Here's how the part is built. I have some questions about the finished solid (model axes, mm). A direction names the side the tool comes from. Give positions to 0.01 mm unless a question says otherwise; leave off trailing zeros. Loops run counter-clockwise (first coordinate to the right, second up) from the corner with the lowest first, then second, coordinate; pieces in that order, holes last. Notation, with made-up numbers: (42, 74) - (87, 74) arc R29 ccw to (87, 112) - close; hole circle Ø2 at (31.25, 61). An arc over 180 degrees is marked (long way). Return JSON: item names as keys, results as strings. Group by question number.
(1) If we section it at A-A (x = -38.5): Please give me the cut outline in (y, z), then the cut area to 3 significant figures.
(2) If we mould it in two halves opening along X, with no side actions, what happens to faces 1 (the flat face through (-19, 17, -96)), 2 (the flat face through (-140, 10, -94)), 3 (the flat face through (-69, 17, -11.5)), 4 (the flat face through (-130, -3, -95))? For each: released by +X, released by -X, zero draft, split by the parting line, or undercut.
(3) For P1, Ø1.5, axis at y = -1.5, z = -88, coming from the +X side; P2, Ø1.8, axis at x = -135, z = -5, coming from the -Y side; P3, Ø5, axis at x = -120.5, z = -8, coming from the -Y side; P4, Ø1.5, axis at y = -1.5, z = -110, coming from the -X side, each with a flat end and sliding along its axis, tell me the tip position at first contact or that it passes through.
(4) If we section it at C-C (y = 5.5): Please give me the cut outline in (x, z).
(5) I need wall thicknesses on probe 1 along X at (y, z) = (6, -5); probe 2 along Z at (x, y) = (-5, 4.25); probe 3 along X at (y, z) = (14.75, -5). Which ranges of each line are inside material? Lowest first, please. Write a range as [from, to].
(6) On a 3-axis mill with a long thin cutter (end or side, diameter ignored), from which of +Z, -Z, +X, -X, +Y, -Y can I reach the whole of each face in a straight line? I mean faces 5 (the flat face through (-71, 6, -185.4)), 6 (the flat face through (-121, 17, -94)), 7 (the flat face through (-133, -1, -183)). Say none if no direction works.
(7) If we section it at B-B (z = -138): Please give me the cut outline in (x, y).
Autodesk Inventor part; units mm, degrees
ref_plane "YZ Plane" through (0, 0, 0) normal (1, 0, 0) x (0, 1, 0)
ref_plane "XZ Plane" through (0, 0, 0) normal (0, 1, 0) x (-1, 0, 0)
ref_plane "XY Plane" through (0, 0, 0) normal (0, 0, 1) x (1, 0, 0)
sketch "Sketch1" plane through (0, 0, 0) normal (0, 1, 0) x (-1, 0, 0)
  line L0 (2, 0) -> (138, 0)
  line L1 (140, -2) -> (140, -188)
  line L2 (138, -190) -> (2, -190)
  line L3 (0, -188) -> (0, -2)
  arc A0 (140, -2) -> (138, 0) centre (138, -2) ccw
  arc A1 (2, 0) -> (0, -2) centre (2, -2) ccw
  arc A2 (0, -188) -> (2, -190) centre (2, -188) ccw
  arc A3 (138, -190) -> (140, -188) centre (138, -188) ccw
  line L4 (21, -11.5) -> (119, -11.5)
  line L5 (121, -13.5) -> (121, -176.5)
  line L6 (119, -178.5) -> (21, -178.5)
  line L7 (19, -176.5) -> (19, -13.5)
  arc A4 (121, -13.5) -> (119, -11.5) centre (119, -13.5) ccw
  arc A5 (119, -178.5) -> (121, -176.5) centre (119, -176.5) ccw
  arc A6 (19, -176.5) -> (21, -178.5) centre (21, -176.5) ccw
  arc A7 (21, -11.5) -> (19, -13.5) centre (21, -13.5) ccw
  point P0 (0, 0)
  point P1 (140, -190)
  point P2 (140, 0)
  point P3 (0, -190)
  point P4 (121, -178.5)
  point P5 (121, -11.5)
  point P6 (19, -178.5)
  dimension "d5" = 190
  dimension "d6" = 140
  dimension "d7" = 102
  dimension "d8" = 167
  dimension "d9" = 2
  dimension "d57" = 11.5
  dimension "d58" = 19
extrude "Extrusion1" add sketch "Sketch1" along normal blind 20
sketch "Sketch2" plane through (0, 0, 0) normal (0, -1, 0) x (1, 0, 0)
  line L0 (-11, -3) -> (-129, -3)
  line L1 (-137, -11) -> (-137, -179)
  line L2 (-129, -187) -> (-11, -187)
  line L3 (-3, -179) -> (-3, -11)
  line L4 (-137, -179) -> (-129, -187)
  line L5 (-137, -11) -> (-129, -3)
  line L6 (-11, -3) -> (-3, -11)
  line L7 (-11, -187) -> (-3, -179)
  line L8 (-129, -187) -> (-129, -185.4)
  line L9 (-129, -185.4) -> (-11, -185.4)
  line L10 (-11, -185.4) -> (-11, -4.6)
  line L11 (-11, -4.6) -> (-129, -4.6)
  line L12 (-129, -4.6) -> (-129, -185.4)
  point P0 (0, 0)
  point P1 (-3, -3)
  point P2 (-137, -187)
  point P3 (-137, -3)
  point P4 (-3, -187)
  dimension "d86" = 134
  dimension "d87" = 184
  dimension "d88" = 8
  dimension "d89" = 8
  dimension "d90" = 8
  dimension "d91" = 8
  dimension "d92" = 8
  dimension "d93" = 8
  dimension "d94" = 8
  dimension "d95" = 8
  dimension "d96" = 1.6
  dimension "d97" = 180.8
  dimension "d98" = 180.8
extrude "Extrusion2" add sketch "Sketch2" along normal blind 3
hole "Hole1" at (-135, 20, -5) direction (0, -1, 0) diameter 3 end through all countersink diameter 5 countersink angle 90
hole "Hole2" at (-135, 20, -185) direction (0, -1, 0) diameter 3 end through all countersink diameter 5 countersink angle 90
hole "Hole3" at (-5, 20, -185) direction (0, -1, 0) diameter 3 end through all countersink diameter 5 countersink angle 90
hole "Hole4" at (-5, 20, -5) direction (0, -1, 0) diameter 3 end through all countersink diameter 5 countersink angle 90
hole "Hole5" at (-120.5, 0, -8) direction (0, 1, 0) diameter 3 depth 19 tip angle 118
hole "Hole6" at (-19.5, 0, -8) direction (0, 1, 0) diameter 3 depth 19 tip angle 118
hole "Hole7" at (-120.5, 0, -182) direction (0, 1, 0) diameter 3 depth 19 tip angle 118
hole "Hole8" at (-19.5, 0, -182) direction (0, 1, 0) diameter 3 depth 19 tip angle 118
sketch "Sketch3" plane through (0, 0, 0) normal (0, -1, 0) x (1, 0, 0)
  line L0 (-11, -185.4) -> (-11, -4.6)
  line L1 (-129, -4.6) -> (-11, -4.6)
  line L2 (-11, -185.4) -> (-129, -185.4)
  line L3 (-129, -185.4) -> (-129, -4.6)
  line L4 (-129, -4.6) -> (-11, -4.6)
  line L5 (-11, -4.6) -> (-11, -185.4)
  point P0 (0, 0)
extrude "Extrusion3" cut sketch "Sketch3" against normal blind 14
properties part number "Dessus boitier"
Values:
{
 "1": {"outline": "(-3, -187) - (0, -187) - (0, -190) - (20, -190) - (20, -178.5) - (14, -178.5) - (14, -185.4) - (-3, -185.4) - close; (-3, -4.6) - (14, -4.6) - (14, -11.5) - (20, -11.5) - (20, 0) - (0, 0) - (0, -3) - (-3, -3) - close", "area": "276 mm2"},
 "2": {"face 1": "undercut", "face 2": "released by -X", "face 3": "undercut", "face 4": "zero draft"},
 "3": {"P1": "x = -3", "P2": "through", "P3": "y = 14", "P4": "x = -137"},
 "4": {"outline": "(-140, -188) arc R2 ccw to (-138, -190) - (-2, -190) arc R2 ccw to (0, -188) - (0, -2) arc R2 ccw to (-2, 0) - (-138, 0) arc R2 ccw to (-140, -2) - close; hole circle Ø3 at (-135, -185); hole circle Ø3 at (-135, -5); hole (-129, -185.4) - (-11, -185.4) - (-11, -4.6) - (-129, -4.6) - close; hole circle Ø3 at (-5, -185); hole circle Ø3 at (-5, -5)"},
 "5": {"probe 1": "[-140, -136.5], [-133.5, -129], [-11, -6.5], [-3.5, 0]", "probe 2": "[-190, -186.5], [-183.5, -6.5], [-3.5, 0]", "probe 3": "[-140, -136.5], [-133.5, -6.5], [-3.5, 0]"},
 "6": {"face 5": "-Y", "face 6": "+Y, -Y", "face 7": "-Z, -X, -Y"},
 "7": {"outline": "(-140, 0) - (-137, 0) - (-137, -3) - (-129, -3) - (-129, 14) - (-121, 14) - (-121, 20) - (-140, 20) - close; (-19, 14) - (-11, 14) - (-11, -3) - (-3, -3) - (-3, 0) - (0, 0) - (0, 20) - (-19, 20) - close"}
}
